```python
from build123d import *

# Parameters (mm, degrees)
BOSS_EXTRU_1_DEPTH      = 2
ESQUISSE2_R             = 3.390627372
ESQUISSE2_R_2           = 1
BOSS_EXTRU_2_DEPTH      = 9.4
ESQUISSE3_R             = 10
ENL_V_MAT_EXTRU_1_DEPTH = 2
BOSS_EXTRU_4_DEPTH      = 5


with BuildPart() as part:
    # Esquisse1 → Boss.-Extru.1 (new body)
    with BuildSketch(Plane(origin=(-56.095259607, 61.741123985, 0), x_dir=(0, 0, 1), z_dir=(0.6724559427452335, -0.7401371528754785, 0))):
        Polygon((-13.170985067, 24.825265138), (-13.170985067, 56.986737001), (-18.722825356, 62.53857729), (-18.722825356, 59.57280759), (-28.570985067, 59.57280759), (-28.570985067, 62.962841359), (-37.970985067, 62.962841359), (-37.970985067, 59.57280759), (-47.970985067, 59.57280759), (-47.970985067, 18.84916078), (-19.147089425, 18.84916078), align=None)
    extrude(amount=-BOSS_EXTRU_1_DEPTH)

    # Esquisse2 → Boss.-Extru.2 (add)
    with BuildSketch(Plane(origin=(0, 0, -37.970985067), x_dir=(-1, 0, 0), z_dir=(0, 0, -1))):
        with Locations((101.983702424, 18.170834722)):
            Circle(ESQUISSE2_R)
        with Locations((101.983702424, 18.170834722)):
            Circle(ESQUISSE2_R_2, mode=Mode.SUBTRACT)
    extrude(amount=-BOSS_EXTRU_2_DEPTH)

    # Esquisse3 → Enlèv. mat.-Extru.1 (cut)
    with BuildSketch(Plane(origin=(-56.095259607, 61.741123985, 0), x_dir=(0, 0, -1), z_dir=(0.6724559427452331, -0.7401371528754788, 0))):
        with Locations(Location((30.570985067, -39.210984185, 0), (0, 0, 90))):
            Circle(ESQUISSE3_R)
    extrude(amount=-ENL_V_MAT_EXTRU_1_DEPTH, mode=Mode.SUBTRACT)

    # Esquisse4 → Boss.-Extru.4 (add)
    with BuildSketch(Plane(origin=(0, 0, -47.970985067), x_dir=(-1, 0, 0), z_dir=(0, 0, -1))):
        with BuildLine():
            Line((73.931199041, 50.400140176), (73.907590469, 51.325240797))
            ThreePointArc((73.907590469, 51.325240797), (74.044969666, 51.682415216), (74.394671882, 51.837833908))
            Line((74.394671882, 51.837833908), (75.194671882, 51.858249912))
            Line((75.194671882, 51.858249912), (75.209983884, 51.258249912))
            Line((75.209983884, 51.258249912), (74.909821146, 51.250589757))
            ThreePointArc((74.909821146, 51.250589757), (74.560118931, 51.095171065), (74.422739734, 50.737996646))
            Line((74.422739734, 50.737996646), (74.499711728, 47.721853148))
            Line((74.499711728, 47.721853148), (73.019437422, 49.066765034))
            Line((73.019437422, 49.066765034), (73.723569144, 49.841766063))
            ThreePointArc((73.723569144, 49.841766063), (73.881297111, 50.10090571), (73.931199041, 50.400140176))
        make_face()
    extrude(amount=-BOSS_EXTRU_4_DEPTH)


solid = part.part
```
Source: CAD feature listing. Evaluate the final solid. Frame: model axes, mm. A direction names the side the tool comes from. Round coordinates to 2 decimals unless told otherwise and drop trailing zeros. Loops run counter-clockwise (first coordinate to the right, second up) from the corner with the lowest first, then second, coordinate; pieces in that order, holes last. Notation, with made-up numbers: M -35,20 L 18,20 A28 ccw 18,47 Z; hole C -19.75,-4 d3. An arc over 180 degrees is marked long. Use a Markdown table: item, result. Add a question column.
1. Cut plane C-C, the plane z = -44.5. Output: boundary loops of the cut face in (x, y).
2. Cut plane B-B, the plane z = -27. Output: boundary loops of the cut face in (x, y), and give its area (3 significant figures).
3. Set-up query: faces 1 (the flat face through (-74.1, 50, -42.971)), 2 (the flat face through (-100.85, 22.41, -42.9)), 3 (the flat face through (-102, 21, -18.723)). Return all of +Z, -Z, +X, -X, +Y, -Y with unobstructed straight access to the full face (end or side cutting, diameter ignored); none if empty.
4. Pull-direction query (X, two-part tool) for faces 4 (the flat face through (-100.962, 22.309, -15.908)), 5 (the cylindrical face through (-102.521, 19.014, -33.337)), 6 (the flat face through (-101, 19, -37.971)), 7 (the flat face through (-72.89, 47.81, -16.2)); classes: +X half, -X half, draft (parallel to the pull), parting line (faces both ways), or undercut.
5. Cut plane A-A, the plane z = -35. State how many separate pieces and enclosed holes the cut face has, and give its area (3 significant figures).
6. Cut plane D-D, the plane x = -95. Output: boundary loops of the cut face in (y, z).
7. Ray query, line 1 along Y through (x, z) = (-99, -21); line 2 along Y through (x, z) = (-99.5, -26); line 3 along X through (y, z) = (38, -16.5). Return the intervals inside material, ascending. Write a range as [from, to].
8. Contact query for flat-ended pins moving along their axis: pin 1 (5 mm diameter, centred on y = 43.5, z = -22.5, fed in from -X); pin 2 (3 mm diameter, centred on y = 43.5, z = -16.5, fed in from -X); pin 3 (5.5 mm diameter, centred on x = -101, y = 20.5, fed in from -Z); pin 4 (2 mm diameter, centred on x = -102, y = 20, fed in from +Z). Output: stop coordinate, or through.
Solution:
| question | item | result |
|---|---|---|
| 1 | outline | M -101.53,23.16 L -100.19,21.68 L -70.05,49.07 L -71.39,50.55 L -73.02,49.07 L -73.72,49.84 A0.8 cw -73.93,50.4 L -73.91,51.33 A0.5 ccw -74.39,51.84 L -75.19,51.86 L -75.21,51.26 L -74.91,51.25 A0.5 cw -74.42,50.74 L -74.5,47.72 Z |
| 2 | outline | M -101.53,23.16 L -100.19,21.68 L -92.03,29.09 L -93.38,30.57 Z; M -79.55,43.13 L -78.2,41.65 L -70.05,49.07 L -71.39,50.55 Z |
| 2 | area | 44.1 mm2 |
| 3 | face 1 | +Z, -X, +Y |
| 3 | face 2 | -Z, -X, -Y |
| 3 | face 3 | -X, -Y |
| 4 | face 4 | -X half |
| 4 | face 5 | undercut |
| 4 | face 6 | draft |
| 4 | face 7 | +X half |
| 5 | separate pieces | 2 |
| 5 | enclosed holes | 1 |
| 5 | area | 81.5 mm2 |
| 6 | outline | M 26.39,-47.97 L 29.1,-47.97 L 29.1,-13.17 L 26.39,-13.17 Z |
| 7 | line 1 | y = [22.76, 25.46] |
| 7 | line 2 | y = [22.31, 25.01] |
| 7 | line 3 | x = [-85.2, -82.23] |
| 8 | pin 1 | stops at x = -81.9 |
| 8 | pin 2 | stops at x = -80.8 |
| 8 | pin 3 | stops at z = -47.97 |
| 8 | pin 4 | stops at z = -17.23 |
